Geometry check sheet. Reference: the model listing, model coordinates, mm. A direction names the side the tool comes from. Coordinates: 2 decimals unless noted, no trailing zeros. Write each loop counter-clockwise with the first axis right and the second up, starting at its lowest first coordinate (ties: lowest second). Pieces come first, ordered by that corner, then holes. Notation, with made-up numbers: (-21, -24) - (21, -24) arc R27 cw to (21, 5) - close; hole circle Ø9 at (-2.75, -25.5). An arc over 180 degrees is marked (long way). Answer as a JSON object with one key per item and string values. Group by question number.
Solid Edge part; units mm, degrees
sketch "Sketch1" plane through (0, 0, 0) normal (0, 0, 1) x (1, 0, 0)
  circle A0 centre (0, 0) radius 2
extrude "Protrusion1" add sketch "Sketch1" along normal blind 10
sketch "Sketch2" plane through (0, 0, 10) normal (0, 0, 1) x (1, 0, 0)
  circle A0 centre (0, 0) radius 4
extrude "Extrusionsausprägung_2" add sketch "Sketch2" along normal blind 3
chamfer "Fase_1" distance 0.5 angle 45 1 edges at (-2, 0, 0)
(1) Material ranges on L1, parallel to Z at x = -2, y = -1.25; L2, parallel to Y at x = 0.5, z = 11.75; L3, parallel to Y at x = -1.75, z = 1.75, recorded low to high. Write a range as [from, to].
(2) Gauge pin test, flat ends, axial feed: pin 1 (2 mm diameter, centred on x = 1.5, z = 8, fed in from -Y); pin 2 (1.5 mm diameter, centred on x = -2, z = 2, fed in from +Y). Record the tip position at first contact, or that the pin passes through.
(3) Set-up check for faces 1 (the face through (0, 0, 13)), 2 (the face through (0, 2, 5)): record each of +Z, -Z, +X, -X, +Y, -Y from which the full face is reachable in a straight line by a thin tool's end or side.
(4) Section check A-A (x = 0). Record the cut outline in (y, z), and give its area (4 significant figures).
(5) Draft check along Y on faces 3 (the face through (0, 0, 0)), 4 (the face through (-0.867, 3.905, 11.479)). Enter one of: +Y half, -Y half, draft (parallel to the pull), parting line (faces both ways), or undercut.
(6) Section check D-D (z = 3.5). Record the cut outline in (x, y).
(7) Section check C-C (z = 11.25). Record the cut outline in (x, y).
Conclusion:
{
 "1": {"L1": "z = [10, 13]", "L2": "y = [-3.97, 3.97]", "L3": "y = [-0.97, 0.97]"},
 "2": {"pin 1": "stops at y = -1.94", "pin 2": "stops at y = 1.56"},
 "3": {"face 1": "+Z, +X, -X, +Y, -Y", "face 2": "-Z"},
 "4": {"outline": "(-4, 10) - (-2, 10) - (-2, 0.5) - (-1.5, 0) - (1.5, 0) - (2, 0.5) - (2, 10) - (4, 10) - (4, 13) - (-4, 13) - close", "area": "63.75 mm^2"},
 "5": {"face 3": "draft", "face 4": "parting line"},
 "6": {"outline": "circle Ø4 at (0, 0)"},
 "7": {"outline": "circle Ø8 at (0, 0)"}
}
